The model under review builds one solid part; all positions refer to its coordinate system, in mm. A direction names the side the tool comes from. Round coordinates to 2 decimals unless told otherwise and drop trailing zeros. Loops run counter-clockwise (first coordinate to the right, second up) from the corner with the lowest first, then second, coordinate; pieces in that order, holes last. Notation, with made-up numbers: M 64,87 L 77,87 A20 cw 77,91 Z; hole C 75,81 d4. An arc over 180 degrees is marked long. Answer as a JSON object with one key per item and string values. Group by question number.
Item 1: Consider section C-C (y = 33). Give the boundary of the cut face in (x, z), and give its area (3 significant figures).
Item 2: Tool access review of faces 1 (the face through (327.14, 99.559, 145.386)), 2 (the face through (346, 131.5, 542)), 3 (the face through (329, 68.5, 542)): name each direction out of +Z, -Z, +X, -X, +Y, -Y from which nothing blocks a thin tool from reaching the whole face with its end or side.
Item 3: To check wall thickness, follow line 1 (X direction, y = 89, z = 150); line 2 (X direction, y = 45, z = 658); line 3 (Y direction, x = 313.5, z = 298). State the ranges of each line that lie inside material, in increasing order.
Item 4: Insertion check: P1, Ø20.5, axis at y = 182, z = 502, coming from the +X side; P2, Ø23, axis at x = 337.5, z = 550, coming from the -Y side. Each pin has a flat end and moves straight along its axis. Give the tip position at first contact, or say it passes through.
Item 5: The part is to be moulded in two halves that separate along Z. For faces 4 (the face through (143, 101, 0)), 5 (the face through (143, 101, 1100)), 6 (the face through (340.5, 99.56, 540.46)), 7 (the face through (300, 34, 542)), say which applies: +Z half, -Z half, draft (parallel to the pull), parting line (faces both ways), or undercut.
Item 6: Consider section B-B (z = 729.5). Give the boundary of the cut face in (x, y).
Item 7: Consider section A-A (z = 550). Give the boundary of the cut face in (x, y).
```python
from build123d import *

# Parameters (mm, degrees)
BOSS_EXTRU_1_DEPTH      = 1100
ENL_V_MAT_EXTRU_1_REACH = 1171.58
ESQUISSE2_R             = 10
ENL_V_MAT_EXTRU_2_REACH = 1171.58
ESQUISSE3_R             = 10


with BuildPart() as part:
    # Esquisse1 → Boss.-Extru.1 (new body)
    with BuildSketch(Plane.XY):
        Polygon((0, 0), (300, 0), (300, 68.5), (375, 68.5), (375, 131.5), (300, 131.5), (300, 200), (0, 200), align=None)
    extrude(amount=BOSS_EXTRU_1_DEPTH)

    # Esquisse2 → Enlèv. mat.-Extru.1 (cut, up to next)
    with BuildSketch(Plane.XZ.offset(-68.5), mode=Mode.PRIVATE) as enl_v_mat_extru_1_sk1:
        with Locations(Location((337.5, 550, 0), (0, 0, 270))):
            Circle(ESQUISSE2_R)
    enl_v_mat_extru_1_tool1 = extrude(enl_v_mat_extru_1_sk1.sketch, amount=-ENL_V_MAT_EXTRU_1_REACH, mode=Mode.PRIVATE) & part.part
    add(enl_v_mat_extru_1_tool1.solids().sort_by_distance((337.5, 68.5, 550))[0], mode=Mode.SUBTRACT)

    # Esquisse3 → Enlèv. mat.-Extru.2 (cut, up to next)
    with BuildSketch(Plane.XZ.offset(-68.5), mode=Mode.PRIVATE) as enl_v_mat_extru_2_sk1:
        with Locations(Location((336.011391588, 150, 0), (0, 0, 270))):
            Circle(ESQUISSE3_R)
    enl_v_mat_extru_2_tool1 = extrude(enl_v_mat_extru_2_sk1.sketch, amount=-ENL_V_MAT_EXTRU_2_REACH, mode=Mode.PRIVATE) & part.part
    add(enl_v_mat_extru_2_tool1.solids().sort_by_distance((336.011392, 68.5, 150))[0], mode=Mode.SUBTRACT)


solid = part.part
```
Geometry results:
{
 "1": {"outline": "M 0,0 L 300,0 L 300,1100 L 0,1100 Z", "area": "330,000 mm^2"},
 "2": {"face 1": "+Y, -Y", "face 2": "+Z, -Z, +X, +Y", "face 3": "+Z, -Z, +X, -Y"},
 "3": {"line 1": "x = 0 to 326.01, 346.01 to 375", "line 2": "x = 0 to 300", "line 3": "y = 68.5 to 131.5"},
 "4": {"P1": "stops at x = 300", "P2": "stops at y = 68.5"},
 "5": {"face 4": "-Z half", "face 5": "+Z half", "face 6": "undercut", "face 7": "draft"},
 "6": {"outline": "M 0,0 L 300,0 L 300,68.5 L 375,68.5 L 375,131.5 L 300,131.5 L 300,200 L 0,200 Z"},
 "7": {"outline": "M 0,0 L 300,0 L 300,68.5 L 327.5,68.5 L 327.5,131.5 L 300,131.5 L 300,200 L 0,200 Z; M 347.5,68.5 L 375,68.5 L 375,131.5 L 347.5,131.5 Z"}
}
